Part model, mm, in its own coordinate system. A direction names the side the tool comes from. Give positions to 0.01 mm unless a question says otherwise; leave off trailing zeros. Order: outer loops, then holes, each group sorted by start corner. A loop starts at its lowest first (then second) coordinate and runs counter-clockwise, first axis right, second up. Notation, with made-up numbers: (-22, -0.5) - (-5, -0.5) arc R27 cw to (-5, 20.5) - close; hole circle Ø8 at (46, 3.5). An arc over 180 degrees is marked (long way). One line per item, written item: value.
```python
from build123d import *

# Parameters (mm, degrees)
SKETCH1_R               = 23.5
BOSS_EXTRUDE1_DEPTH     = 7
SKETCH2_R               = 17.5
CUT_EXTRUDE1_DEPTH      = 34.963215395
SKETCH3_R               = 22
SKETCH3_R_2             = 19
CUT_EXTRUDE_THIN1_DEPTH = 34.963215395
EXTRUDE_THIN1_START     = 1
SKETCH4_R               = 22
SKETCH4_R_2             = 19
EXTRUDE_THIN1_DEPTH     = 5


with BuildPart() as part:
    # Sketch1 → Boss-Extrude1 (new body)
    with BuildSketch(Plane(origin=(0, 0, 0), x_dir=(0, 1, 0), z_dir=(0, 0, 1))):
        with Locations(Location((0, 0, 0), (0, 0, 270))):
            Circle(SKETCH1_R)
    extrude(amount=BOSS_EXTRUDE1_DEPTH)

    # Sketch2 → Cut-Extrude1 (cut, through all)
    with BuildSketch(Plane(origin=(0, 0, 0), x_dir=(0, 1, 0), z_dir=(0, 0, 1))):
        with Locations(Location((0, 0, 0), (0, 0, 270))):
            Circle(SKETCH2_R)
    extrude(amount=CUT_EXTRUDE1_DEPTH, mode=Mode.SUBTRACT)

    # Sketch3 → Cut-Extrude-Thin1 (cut, through all)
    with BuildSketch(Plane(origin=(0, 0, 0), x_dir=(1, 0, 0), z_dir=(0, 0, -1))):
        Circle(SKETCH3_R)
        Circle(SKETCH3_R_2, mode=Mode.SUBTRACT)
    extrude(amount=-CUT_EXTRUDE_THIN1_DEPTH, mode=Mode.SUBTRACT)


with BuildPart() as cut_extrude_thin1_piece_1:
    # of the separate pieces the step leaves, piece 1, a body of its own (cut_extrude_thin1_pieces)
    add(part.part.solids().sort_by_distance((23.5, 0, 0))[0])



with BuildPart() as cut_extrude_thin1_piece_2:
    # of the separate pieces the step leaves, piece 2, a body of its own (cut_extrude_thin1_pieces)
    add(part.part.solids().sort_by_distance((19, 0, 0))[0])


with BuildPart() as cut_extrude_thin1_piece_1_1:
    add(cut_extrude_thin1_piece_1.part)

    add(cut_extrude_thin1_piece_2.part)  # Extrude-Thin1 merges Cut-Extrude-Thin1 piece 2
    # Sketch4 → Extrude-Thin1 (add)
    with BuildSketch(Plane(origin=(0, 0, 0), x_dir=(0, 1, 0), z_dir=(0, 0, 1)).offset(EXTRUDE_THIN1_START)):
        Circle(SKETCH4_R)
        Circle(SKETCH4_R_2, mode=Mode.SUBTRACT)
    extrude(amount=EXTRUDE_THIN1_DEPTH)


solid = cut_extrude_thin1_piece_1_1.part
```
1) Mould opens along Y. For faces 1 (the cylindrical face through (-17.32, 15.88, 3.45)), 2 (the cylindrical face through (18.12, -5.71, 0.49)), 3 (the flat face through (6, -17, 0)) say: released by +Y, released by -Y, zero draft, split by the parting line, or undercut.
Outcome:
face 1: split by the parting line
face 2: undercut
face 3: zero draft
2) Cut at C-C, the plane z = 3.25. Give the cut face in (x, y), then the cut area to 3 significant figures.
Outcome:
outline: circle Ø47 at (0, 0); hole circle Ø35 at (0, 0)
area: 773 mm^2
3) Which spindle directions (+Z, -Z, +X, -X, +Y, -Y) get a long thin tool onto all of the face, cutting with end or side? Do faces 4 (the flat face through (-18, -7, 6)), 5 (the flat face through (16, -16, 0)), 6 (the cylindrical face through (20.32, 8.43, 0.49)). Say none if no direction does.
Outcome:
face 4: +Z
face 5: -Z, +X, -X, +Y, -Y
face 6: -Z
4) Pin check, flat tip, straight feed: pin 1 (4 mm diameter, centred on x = 11.5, z = 1.5, fed in from -Y). Stop position of the tip, or through.
Outcome:
pin 1: stops at y = -21.49
5) Cut at B-B, the plane y = 15. Give the cut face in (x, z), then the cut area to 3 significant figures.
Outcome:
outline: (-18.09, 0) - (-16.09, 0) - (-16.09, 1) - (-11.66, 1) - (-11.66, 0) - (-9.01, 0) - (-9.01, 7) - (-11.66, 7) - (-11.66, 6) - (-16.09, 6) - (-16.09, 7) - (-18.09, 7) - close; (9.01, 0) - (11.66, 0) - (11.66, 1) - (16.09, 1) - (16.09, 0) - (18.09, 0) - (18.09, 7) - (16.09, 7) - (16.09, 6) - (11.66, 6) - (11.66, 7) - (9.01, 7) - close
area: 109 mm^2
6) Drill centre lines: line 1 along Y through (x, z) = (0, 6.5); line 2 along X through (y, z) = (4.5, 6.5); line 3 along X through (y, z) = (-3, 5.25). Where is each one in solid material? Low to high. Write a range as from..to.
Outcome:
line 1: y = -23.5..-22, -19..-17.5, 17.5..19, 22..23.5
line 2: x = -23.07..-21.53, -18.46..-16.91, 16.91..18.46, 21.53..23.07
line 3: x = -23.31..-17.24, 17.24..23.31
7) Cut at D-D, the plane y = 20. Give the cut face in (x, z).
Outcome:
outline: (-12.34, 0) - (-9.17, 0) - (-9.17, 1) - (9.17, 1) - (9.17, 0) - (12.34, 0) - (12.34, 7) - (9.17, 7) - (9.17, 6) - (-9.17, 6) - (-9.17, 7) - (-12.34, 7) - close
8) Cut at A-A, the plane x = 0. Give the cut face in (y, z), then the cut area to 3 significant figures.
Outcome:
outline: (-23.5, 0) - (-22, 0) - (-22, 1) - (-19, 1) - (-19, 0) - (-17.5, 0) - (-17.5, 7) - (-19, 7) - (-19, 6) - (-22, 6) - (-22, 7) - (-23.5, 7) - close; (17.5, 0) - (19, 0) - (19, 1) - (22, 1) - (22, 0) - (23.5, 0) - (23.5, 7) - (22, 7) - (22, 6) - (19, 6) - (19, 7) - (17.5, 7) - close
area: 72.0 mm^2
